Geometry check sheet. Reference: the model listing, model coordinates, mm. A direction names the side the tool comes from. Round coordinates to 2 decimals unless told otherwise and drop trailing zeros. Order: outer loops, then holes, each group sorted by start corner. A loop starts at its lowest first (then second) coordinate and runs counter-clockwise, first axis right, second up. Notation, with made-up numbers: (43, 77.5) - (55, 77.5) arc R32 ccw to (55, 111.5) - close; hole circle Ø10 at (4, 6.5). An arc over 180 degrees is marked (long way). Return JSON: item names as keys, results as strings. Group by question number.
Q1. Sectioned sample at A-A, the plane x = -10. Record the cut outline in (y, z).
Q2. Sectioned sample at B-B, the plane x = 12.5. Record the cut outline in (y, z).
Q3. Tool access check on faces 4 (the flat face through (16, 12, -19.843)), 5 (the flat face through (-8, 13.5, -22)), 6 (the flat face through (-8.73, 11, -23)), 7 (the cylindrical face through (16.193, 4.566, -4.519)), 8 (the cylindrical face through (16.193, 1.087, -11.941)). Record the directions out of +Z, -Z, +X, -X, +Y, -Y that give a thin tool (end or side, any length) a straight path to the whole face; none if there is none.
Q4. Gauge pin test, flat ends, axial feed: pin 1 Ø0.6 at (x, z) = (-7.5, -22) entering from -Y; pin 2 Ø3 at (y, z) = (10.5, 0) entering from -X; pin 3 Ø2 at (x, y) = (1.5, 7) entering from -Z; pin 4 Ø12 at (x, z) = (-4.5, 12.5) entering from +Y. Record the tip position at first contact, or that the pin passes through.
Q5. Draft check along Y on faces 1 (the flat face through (-22.73, 12, 10)), 2 (the flat face through (-2, 8.784, -22)), 3 (the flat face through (-6.73, 10, -21)). Enter one of: pulls with the +Y half, pulls with the -Y half, needs draft (parallel to the pull), parting line crosses it, or undercut.
Q6. Sectioned sample at C-C, the plane z = 16.5. Record the cut outline in (x, y), then the cut area to 3 significant figures.
Q7. Material ranges on line 1 along Z through (x, y) = (7.5, 12.5); line 2 along X through (y, z) = (21.75, -3); line 3 along Z through (x, y) = (-4, 16.25), recorded low to high.
```python
from build123d import *

# Parameters (mm, degrees)
SKETCH1_W                = 14
SKETCH1_H                = 42
MAIN_BODY_DEPTH          = 23
FILLET1_R                = 2
MOTOR_HOLDER_DEPTH       = 18.5
BOSS_EXTRUDE3_DEPTH      = 5
SKETCH4_R                = 1.1
NUT_HOLES_DEPTH          = 15
SKETCH5_W                = 2
SKETCH5_H                = 4
BOSS_EXTRUDE4_DEPTH      = 5
BOSS_EXTRUDE5_DEPTH      = 4
CUT_EXTRUDE2_DEPTH       = 2
BOSS_EXTRUDE6_DEPTH      = 14
BOSS_EXTRUDE7_DEPTH      = 2
FILLET2_R                = 3
BOSS_EXTRUDE8_DEPTH      = 2.2
BOSS_EXTRUDE8_DEPTH_BACK = 2.2
FILLET3_R                = 1
SKETCH12_R               = 3.5
SKETCH12_R_2             = 3.070336519
BOSS_EXTRUDE9_DEPTH      = 1
SKETCH14_R               = 3
BOSS_EXTRUDE10_DEPTH     = 1
SKETCH15_R               = 1
SHAFT_DEPTH              = 7
SKETCH16_R               = 2
BOSS_EXTRUDE12_DEPTH     = 1.5


with BuildPart() as part:
    # Sketch1 → Main Body (new body)
    with BuildSketch(Plane(origin=(0, 0, 0), x_dir=(1, 0, 0), z_dir=(0, 1, 0))):
        with Locations((-14.72963025, -0.456790856)):
            Rectangle(SKETCH1_W, SKETCH1_H)
    extrude(amount=MAIN_BODY_DEPTH)

    # Fillet1
    fillet1_edges = [part.edges().sort_by_distance(p)[0] for p in [
        (-14.72963025, 23, -20.543209144),
        (-14.72963025, 0, -20.543209144),
        (-14.72963025, 0, 21.456790856),
        (-14.72963025, 23, 21.456790856),
    ]]
    fillet(fillet1_edges, radius=FILLET1_R)

    # Sketch2 → Motor Holder (add)
    with BuildSketch(Plane(origin=(-7.72963025, 0, 0), x_dir=(0, 0, -1), z_dir=(1, 0, 0))):
        with BuildLine():
            Line((3.543209144, 19.033283793), (3.543209144, 3.966716207))
            ThreePointArc((3.543209144, 3.966716207), (12.043209144, 0.142167253), (20.543209144, 3.966716207))
            Line((20.543209144, 3.966716207), (20.543209144, 19.033283793))
            ThreePointArc((20.543209144, 19.033283793), (12.043209144, 22.857832747), (3.543209144, 19.033283793))
        make_face()
    extrude(amount=MOTOR_HOLDER_DEPTH)

    # Sketch3 → Boss-Extrude3 (add)
    with BuildSketch(Plane(origin=(-7.72963025, 0, 0), x_dir=(0, 0, -1), z_dir=(1, 0, 0))):
        with BuildLine():
            Line((3.543209144, 12.866872794), (3.543209144, 10.327683852))
            ThreePointArc((3.543209144, 10.327683852), (3.130583543, 10.726570697), (2.605351044, 10.495266949))
            ThreePointArc((2.605351044, 10.495266949), (-1.12344994, 11.454900344), (2.558290761, 12.581682682))
            ThreePointArc((2.558290761, 12.581682682), (3.155784465, 12.361535772), (3.543209144, 12.866872794))
        make_face()
    extrude(amount=BOSS_EXTRUDE3_DEPTH)

    # Sketch4 → Nut Holes (cut)
    with BuildSketch(Plane(origin=(-7.72963025, 0, 0), x_dir=(0, 0, -1), z_dir=(1, 0, 0))):
        with Locations((-18.956790856, 20.5)):
            Circle(SKETCH4_R)
        with Locations((-18.956790856, 2.5)):
            Circle(SKETCH4_R)
    extrude(amount=-NUT_HOLES_DEPTH, mode=Mode.SUBTRACT)

    # Sketch5 → Boss-Extrude4 (add)
    with BuildSketch(Plane(origin=(0, 0, -20.543209144), x_dir=(-1, 0, 0), z_dir=(0, 0, -1))):
        with Locations((7.72963025, 11.5)):
            Rectangle(SKETCH5_W, SKETCH5_H)
    extrude(amount=BOSS_EXTRUDE4_DEPTH)

    # Sketch6 → Boss-Extrude5 (add)
    with BuildSketch(Plane(origin=(-6.72963025, 0, 0), x_dir=(0, 0, -1), z_dir=(1, 0, 0))):
        with BuildLine():
            ThreePointArc((21.679339079, 10.774749435), (23.912167048, 9.534327071), (25.543209144, 11.5))
            ThreePointArc((25.543209144, 11.5), (23.912167048, 13.465672929), (21.679339079, 12.225250565))
            ThreePointArc((21.679339079, 12.225250565), (21.665841795, 12.183376686), (21.649262587, 12.142624651))
            ThreePointArc((21.649262587, 12.142624651), (21.543692429, 11.456035136), (21.679339079, 10.774749435))
        make_face()
        with BuildLine():
            ThreePointArc((20.543209144, 10.774749435), (21.111274111, 11.147288257), (21.679339079, 10.774749435))
            ThreePointArc((21.679339079, 10.774749435), (21.543692429, 11.456035136), (21.649262587, 12.142624651))
            ThreePointArc((21.649262587, 12.142624651), (21.067309248, 11.796717861), (20.543209144, 12.225250565))
            Line((20.543209144, 12.225250565), (20.543209144, 10.774749435))
        make_face()
    extrude(amount=BOSS_EXTRUDE5_DEPTH)

    # Sketch7 → Cut-Extrude2 (cut)
    with BuildSketch(Plane(origin=(-6.72963025, 0, 0), x_dir=(0, 0, -1), z_dir=(1, 0, 0))):
        with BuildLine():
            Line((23.543209144, 13.5), (23.543209144, 13.967200788))
            Line((23.543209144, 13.967200788), (25.760178749, 13.967200788))
            Line((25.760178749, 13.967200788), (25.760178749, 8.970470958))
            Line((25.760178749, 8.970470958), (23.543209144, 8.970470958))
            Line((23.543209144, 8.970470958), (23.543209144, 9.5))
            ThreePointArc((23.543209144, 9.5), (25.543209144, 11.5), (23.543209144, 13.5))
        make_face()
    extrude(amount=-CUT_EXTRUDE2_DEPTH, mode=Mode.SUBTRACT)

    # Sketch8 → Boss-Extrude6 (add)
    with BuildSketch(Plane(origin=(10.77036975, 0, 0), x_dir=(0, 0, -1), z_dir=(1, 0, 0))):
        with BuildLine():
            Line((4.243209144, 17.35646316), (4.243209144, 5.822511997))
            ThreePointArc((4.243209144, 5.822511997), (4.526819665, 4.549237399), (5.324027945, 3.516705516))
            ThreePointArc((5.324027945, 3.516705516), (12.043209144, 1.086287771), (18.762390342, 3.516705516))
            ThreePointArc((18.762390342, 3.516705516), (19.559598622, 4.549237399), (19.843209144, 5.822511997))
            Line((19.843209144, 5.822511997), (19.843209144, 17.35646316))
            ThreePointArc((19.843209144, 17.35646316), (19.559598622, 18.629737758), (18.762390342, 19.66226964))
            ThreePointArc((18.762390342, 19.66226964), (12.043209144, 22.092687386), (5.324027945, 19.66226964))
            ThreePointArc((5.324027945, 19.66226964), (4.526819665, 18.629737758), (4.243209144, 17.35646316))
        make_face()
    extrude(amount=BOSS_EXTRUDE6_DEPTH)

    # Sketch9 → Boss-Extrude7 (add)
    with BuildSketch(Plane(origin=(-2.72963025, 0, 0), x_dir=(0, 0, -1), z_dir=(1, 0, 0))):
        with BuildLine():
            Line((20.534219475, 8.784213792), (23.432322776, 8.784213792))
            Line((23.432322776, 8.784213792), (23.432322776, 9.263820028))
            ThreePointArc((23.432322776, 9.263820028), (25.790969288, 11.48725138), (23.432322776, 13.710682731))
            Line((23.432322776, 13.710682731), (23.432322776, 14.220655847))
            Line((23.432322776, 14.220655847), (20.534219475, 14.220655847))
            Line((20.534219475, 14.220655847), (20.534219475, 8.784213792))
        make_face()
        with BuildLine():
            Line((3.543209144, 8.784213792), (0.645105842, 8.784213792))
            Line((0.645105842, 8.784213792), (0.645105842, 9.294186907))
            ThreePointArc((0.645105842, 9.294186907), (-1.71354067, 11.517618258), (0.645105842, 13.74104961))
            Line((0.645105842, 13.74104961), (0.645105842, 14.220655847))
            Line((0.645105842, 14.220655847), (3.543209144, 14.220655847))
            Line((3.543209144, 14.220655847), (3.543209144, 8.784213792))
        make_face()
    extrude(amount=BOSS_EXTRUDE7_DEPTH)

    # Fillet2
    fillet2_edges = [part.edges().sort_by_distance(p)[0] for p in [
        (24.77036975, 18.629737758, -4.526819665),
        (24.77036975, 11.589487578, -4.243209144),
        (24.77036975, 4.549237399, -4.526819665),
        (24.77036975, 1.086287771, -12.043209144),
        (24.77036975, 4.549237399, -19.559598622),
        (24.77036975, 11.589487578, -19.843209144),
        (24.77036975, 18.629737758, -19.559598622),
        (24.77036975, 22.092687386, -12.043209144),
    ]]
    fillet(fillet2_edges, radius=FILLET2_R)

    # Sketch10 → Boss-Extrude8 (add, two sides)
    with BuildSketch(Plane(origin=(0, 11.5176, 0), x_dir=(1, 0, 0), z_dir=(0, 1, 0))) as boss_extrude8_sk:
        with BuildLine():
            Line((-0.72963025, 21.98776596), (10.910253109, 21.98776596))
            Line((10.910253109, 21.98776596), (24.77036975, 20.809448862))
            ThreePointArc((24.77036975, 20.809448862), (25.391050954, 20.50205534), (25.604727399, 19.843209144))
            Line((25.604727399, 19.843209144), (25.604727399, 4.166099851))
            ThreePointArc((25.604727399, 4.166099851), (25.476560723, 3.537376336), (24.938530753, 3.187742664))
            Line((24.938530753, 3.187742664), (10.910253109, 2.094157493))
            Line((10.910253109, 2.094157493), (-0.72963025, 2.094157493))
            Line((-0.72963025, 2.094157493), (-0.72963025, 3.0856238))
            Line((-0.72963025, 3.0856238), (10.910253109, 3.0856238))
            Line((10.910253109, 3.0856238), (24.77036975, 4.166099851))
            Line((24.77036975, 4.166099851), (24.77036975, 19.843209144))
            Line((24.77036975, 19.843209144), (10.910253109, 21.021526241))
            Line((10.910253109, 21.021526241), (-0.72963025, 21.021526241))
            Line((-0.72963025, 21.021526241), (-0.72963025, 21.98776596))
        make_face()
    extrude(amount=BOSS_EXTRUDE8_DEPTH)
    extrude(boss_extrude8_sk.sketch, amount=-BOSS_EXTRUDE8_DEPTH_BACK)

    # Fillet3
    fillet3_edges = [part.edges().sort_by_distance(p)[0] for p in [
        (-0.72963025, 11.5176, -21.98776596),
        (-0.72963025, 11.5176, -2.094157493),
    ]]
    fillet(fillet3_edges, radius=FILLET3_R)

    # Sketch12 → Boss-Extrude9 (add)
    with BuildSketch(Plane.ZY.offset(21.72963025)):
        with Locations((10.456790856, 11.5)):
            Circle(SKETCH12_R)
        with Locations((10.456790856, 11.5)):
            Circle(SKETCH12_R_2, mode=Mode.SUBTRACT)
    extrude(amount=BOSS_EXTRUDE9_DEPTH)

    # Sketch14 → Boss-Extrude10 (add)
    with BuildSketch(Plane.ZY.offset(21.72963025)):
        with Locations((10.456790856, 11.5)):
            Circle(SKETCH14_R)
    extrude(amount=BOSS_EXTRUDE10_DEPTH)

    # Sketch15 → Shaft (add)
    with BuildSketch(Plane.ZY.offset(22.72963025)):
        with BuildLine():
            Line((8.848293419, 8.967661951), (8.848293419, 14.032338049))
            ThreePointArc((8.848293419, 14.032338049), (10.456790856, 14.5), (12.065288294, 14.032338049))
            Line((12.065288294, 14.032338049), (12.065288294, 8.967661951))
            ThreePointArc((12.065288294, 8.967661951), (10.456790856, 8.5), (8.848293419, 8.967661951))
        make_face()
        with Locations((10.456790856, 11.5)):
            Circle(SKETCH15_R, mode=Mode.SUBTRACT)
    extrude(amount=SHAFT_DEPTH)

    # Sketch16 → Boss-Extrude12 (add)
    with BuildSketch(Plane.ZY.offset(21.72963025)):
        with Locations((-0.543209144, 11.5)):
            Circle(SKETCH16_R)
    extrude(amount=BOSS_EXTRUDE12_DEPTH)


solid = part.part
```
Reply:
{
 "1": {"outline": "(0, -18.54) arc R2 ccw to (2, -20.54) - (21, -20.54) arc R2 ccw to (23, -18.54) - (23, 19.46) arc R2 ccw to (21, 21.46) - (2, 21.46) arc R2 ccw to (0, 19.46) - close; hole circle Ø2.2 at (2.5, 18.96); hole circle Ø2.2 at (20.5, 18.96)"},
 "2": {"outline": "(3.52, -18.76) arc R3 ccw to (5.82, -19.84) - (17.36, -19.84) arc R3 ccw to (19.66, -18.76) arc R10.5 ccw to (19.66, -5.32) arc R3 ccw to (17.36, -4.24) - (5.82, -4.24) arc R3 ccw to (3.52, -5.32) arc R10.5 ccw to start; (9.32, -21.85) - (13.72, -21.85) - (13.72, -20.89) - (9.32, -20.89) - close; (9.32, -3.21) - (13.72, -3.21) - (13.72, -2.22) - (9.32, -2.22) - close"},
 "3": {"face 4": "+Y, -Y", "face 5": "-Z, -X, +Y", "face 6": "-Z, -X, +Y, -Y", "face 7": "+Z, +X, -Y", "face 8": "+X, -Y"},
 "4": {"pin 1": "y = 9.5", "pin 2": "x = -23.23", "pin 3": "z = -20.54", "pin 4": "y = 23"},
 "5": {"face 1": "undercut", "face 2": "pulls with the -Y half", "face 3": "needs draft"},
 "6": {"outline": "(-21.73, 0) - (-7.73, 0) - (-7.73, 23) - (-21.73, 23) - close", "area": "322 mm^2"},
 "7": {"line 1": "-21.99 to -21.02, -20.54 to -3.54, -3.09 to -2.09", "line 2": "-21.73 to -7.73", "line 3": "-20.54 to -3.54"}
}
